Here's how the part is built. I have some questions about the finished solid (model axes, mm). Coordinates: 2 decimals unless noted, no trailing zeros. Write each loop counter-clockwise with the first axis right and the second up, starting at its lowest first coordinate (ties: lowest second). Pieces come first, ordered by that corner, then holes. Notation, with made-up numbers: M -38.5,77.5 L -21.5,77.5 A32 ccw -21.5,107.5 Z; hole C 47,86 d11. An arc over 180 degrees is marked long. Use a Markdown table: item, result.
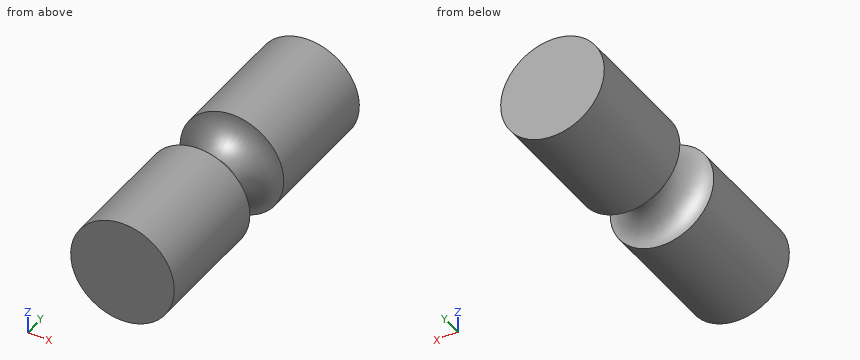
```python
from build123d import *

# Parameters (mm, degrees)
SKETCH1_R           = 10
BOSS_EXTRUDE1_DEPTH = 30


# Read off the part's stored shape, not the designer's step: Cut-Sweep5
with BuildPart() as part:
    # Sketch1 → Boss-Extrude1 (new body)
    with BuildSketch(Plane(origin=(0, 0, 0), x_dir=(1, 0, 0), z_dir=(0, 1, 0))):
        with Locations(Location((0, 0, 0), (0, 0, 270))):
            Circle(SKETCH1_R)
    extrude(amount=BOSS_EXTRUDE1_DEPTH)

    # Cut-Sweep5 outline → Cut-Sweep5 (revolve, cut)
    with BuildSketch(Plane.XY):
        with BuildLine():
            Line((10, 30), (4.5, 30))
            ThreePointArc((4.5, 30), (6.110912703, 26.110912703), (10, 24.5))
            Line((10, 24.5), (10, 30))
        make_face()
    revolve(axis=Axis((0, 0, 0), (0, 1, 0)), mode=Mode.SUBTRACT)

    # Mirror1: part across plane


with BuildPart() as part_1:
    add(part.part)
    add(part.part.mirror(Plane.ZX.offset(30)))


solid = part_1.part
```
1. I need wall thicknesses on probe 1 along Z at (x, y) = (0.5, 14); probe 2 along Y at (x, z) = (7.5, -1); probe 3 along Y at (x, z) = (-1.5, -7.25). Which ranges of each line are inside material? Lowest first, please.
Answers follow:
| item | result |
|---|---|
| probe 1 | z = -9.99 to 9.99 |
| probe 2 | y = 0 to 25.07, 34.93 to 60 |
| probe 3 | y = 0 to 25.15, 34.85 to 60 |
2. Will these pins go through, and if not, where does the flat tip stop? pin 1 Ø10 at (x, y) = (6.5, 22) entering from +Z; pin 2 Ø1.5 at (x, y) = (-1.5, 12.5) entering from +Z; pin 3 Ø4 at (y, z) = (9, 7.5) entering from -X.
Answers follow:
| item | result |
|---|---|
| pin 1 | stops at z = 9.89 |
| pin 2 | stops at z = 9.97 |
| pin 3 | stops at x = -8.35 |
3. Suppose I cut it at B-B on y = 32.5. Write out the boundary of the cut face in (x, z).
Answers follow:
| item | result |
|---|---|
| outline | C 0,0 d10.2 |
4. Suppose I cut it at A-A on y = 53.5. Write out the boundary of the cut face in (x, z).
Answers follow:
| item | result |
|---|---|
| outline | C 0,0 d20 |
